Input: part model. Units: mm. Frame: model coordinates. Face numbers are marked on the shaded views. Coordinates: 2 decimals unless noted, no trailing zeros. Loops run counter-clockwise (first coordinate to the right, second up) from the corner with the lowest first, then second, coordinate; pieces in that order, holes last.
Item 1: Section D-D on y = 19.5. Return loops of the section in (x, z), and give its area (3 significant figures).
Item 2: Section A-A on y = 8.4. Return loops of the section in (x, z), and give its area (3 significant figures).
Item 3: Section B-B on z = 0. Return loops of the section in (x, y), and give its area (3 significant figures).
Item 4: Section C-C on x = -2. Return loops of the section in (y, z), and give its area (3 significant figures).
Item 5: Contact query for flat-ended pins moving along their axis: P1, Ø6, axis at y = 6, z = 4, coming from the -X side; P2, Ø5, axis at x = -16, y = 28, coming from the +Z side; P3, Ø6, axis at x = -5.5, y = 5, coming from the +Z side. Output: stop coordinate, or through.
Item 6: Pull-direction query (Y, two-part tool) for the marked faces 1, 2 and 3; classes: released by +Y, released by -Y, zero draft, split by the parting line, or undercut.
Item 7: Ray query, line 1 along Y through (x, z) = (-16, -5); line 2 along Z through (x, y) = (0, 10.5); line 3 along X through (y, z) = (28.5, 0.75). Return the intervals inside material, ascending.
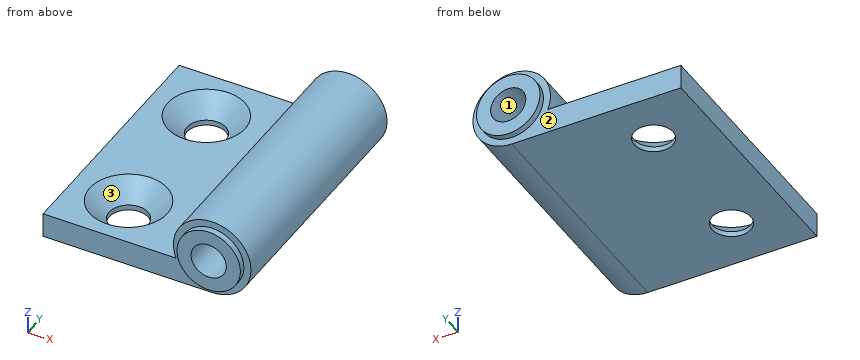
```python
from build123d import *

# Parameters (mm, degrees)
EXTRUDE1_DEPTH      = 35
SKETCH2_W           = 4.5
SKETCH2_H           = 0.9
SKETCH3_W           = 4.5
SKETCH3_H           = 0.9
HOLEWZD1_AT_2_COUNT = 2
HOLEWZD1_AT_2_PITCH = 20
HOLEWZD2_D          = 5
HOLEWZD2_DEPTH      = 36.8


with BuildPart() as part:
    # Sketch1 → Extrude1 (new body)
    with BuildSketch(Plane(origin=(0, 35.9, 0), x_dir=(1, 0, 0), z_dir=(0, 1, 0))):
        with BuildLine():
            Line((-24, 5.5), (-24, 2))
            Line((-24, 2), (-5.123475383, 2))
            ThreePointArc((-5.123475383, 2), (3.102418411, -4.541475531), (0, 5.5))
            Line((0, 5.5), (-24, 5.5))
        make_face()
    extrude(amount=-EXTRUDE1_DEPTH)

    # Sketch2 → Revolve1 (revolve)
    with BuildSketch(Plane.XY):
        with Locations((2.25, 0.45)):
            Rectangle(SKETCH2_W, SKETCH2_H)
    revolve(axis=Axis((0, 0.9, 0), (0, -1, 0)))

    # Sketch3 → Revolve2 (revolve)
    with BuildSketch(Plane.XY):
        with Locations((2.25, 36.35)):
            Rectangle(SKETCH3_W, SKETCH3_H)
    revolve(axis=Axis((0, 36.8, 0), (0, -1, 0)))

    # Sketch4 → HoleWzd1 (revolve, cut)
    with BuildSketch(Plane(origin=(-16, 28.4, -2), x_dir=(0, -1, 0), z_dir=(1, 0, 0))):
        Polygon((0, 0), (0, 3.5), (2.75, 3.5), (2.75, 2.75), (5.5, 0), align=None)
    holewzd1 = revolve(axis=Axis((-16, 28.4, 4.35), (0, 0, -1)), mode=Mode.SUBTRACT)

    # HoleWzd1 at 2: HoleWzd1 ×2
    with Locations(*[(0, -i * HOLEWZD1_AT_2_PITCH, 0) for i in range(1, HOLEWZD1_AT_2_COUNT)]):
        add(holewzd1, mode=Mode.SUBTRACT)

    # HoleWzd2
    with Locations(Plane(origin=(0, 36.8, 0), x_dir=(1, 0, 0), z_dir=(0, 1, 0))):
        with Locations((0, 0)):
            Hole(HOLEWZD2_D / 2, depth=HOLEWZD2_DEPTH)


solid = part.part
```
Results found:
1. outline: (-24, -5.5) - (0, -5.5) arc R5.5 ccw (long way) to (-5.12, -2) - (-24, -2) - close; hole circle Ø5 at (0, 0)
1. area: 146 mm2
2. outline: (-24, -5.5) - (-18.75, -5.5) - (-18.75, -4.75) - (-21.5, -2) - (-24, -2) - close; (-13.25, -5.5) - (0, -5.5) arc R5.5 ccw (long way) to (-5.12, -2) - (-10.5, -2) - (-13.25, -4.75) - close; hole circle Ø5 at (0, 0)
2. area: 120 mm2
3. outline: (-5.5, 0.9) - (-4.5, 0.9) - (-4.5, 0) - (-2.5, 0) - (-2.5, 36.8) - (-4.5, 36.8) - (-4.5, 35.9) - (-5.5, 35.9) - close; (2.5, 0) - (4.5, 0) - (4.5, 0.9) - (5.5, 0.9) - (5.5, 35.9) - (4.5, 35.9) - (4.5, 36.8) - (2.5, 36.8) - close
3. area: 217 mm2
4. outline: (0, -4.03) - (0.9, -4.03) - (0.9, -5.5) - (35.9, -5.5) - (35.9, -4.03) - (36.8, -4.03) - (36.8, -1.5) - (0, -1.5) - close; (0, 1.5) - (36.8, 1.5) - (36.8, 4.03) - (35.9, 4.03) - (35.9, 5.12) - (0.9, 5.12) - (0.9, 4.03) - (0, 4.03) - close
4. area: 276 mm2
5. P1: stops at x = -5.41
5. P2: stops at z = -4.6
5. P3: stops at z = 4.9
6. face 1: zero draft
6. face 2: released by +Y
6. face 3: undercut
7. line 1: y = 0.9 to 5.65, 11.15 to 25.65, 31.15 to 35.9
7. line 2: z = -5.5 to -2.5, 2.5 to 5.5
7. line 3: x = -5.45 to -2.38, 2.38 to 5.45
